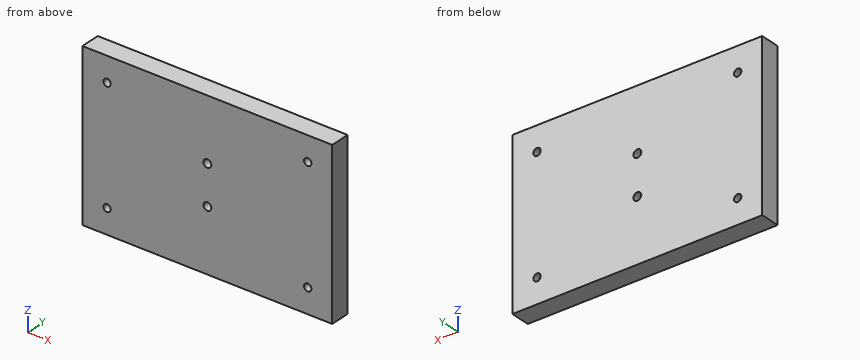
```python
from build123d import *

# Parameters (mm, degrees)
F0_W     = 101.69682
F0_H     = 66.800862
F1_DEPTH = 4
F3_D     = 3
F4_D     = 3.2


with BuildPart() as f1:
    # F0 (on Front) → F1 (new body, symmetric)
    with BuildSketch(Plane.XZ):
        Rectangle(F0_W, F0_H)
    extrude(amount=F1_DEPTH, both=True)

    # F3 (through all)
    with Locations(Plane.XZ.offset(4)):
        with Locations((-40.84841, 23.400431), (40.84841, 23.400431), (40.84841, -23.400431), (-40.84841, -23.400431)):
            Hole(F3_D / 2)

    # F4 (through all)
    with Locations(Plane.XZ.offset(4)):
        with Locations((0, 8), (0, -8)):
            Hole(F4_D / 2)


solid = f1.part
```
Input: part model. Units: mm. Frame: model coordinates. Coordinates: 2 decimals unless noted, no trailing zeros. Loops run counter-clockwise (first coordinate to the right, second up) from the corner with the lowest first, then second, coordinate; pieces in that order, holes last. Notation, with made-up numbers: M -37.75,27 L 14.25,27 A23 ccw 14.25,46 Z; hole C 73,-34 d5. An arc over 180 degrees is marked long. Use a Markdown table: item, result. Add a question column.
1) Section B-B, the plane x = 0. Return the cut outline in (y, z).
2) Line query: L1, parallel to Z at x = 0, y = 2; L2, parallel to X at y = 2, z = 23; L3, parallel to X at y = 3.5, z = -7. Output: solid intervals per line, ascending. Write a range as from..to.
3) Section A-A, the plane z = 8. Return the cut outline in (x, y).
4) Pin query (flat end, axial travel): P1, Ø3.5, axis at x = 0, z = 8, coming from the +Y side. Return the tip coordinate at first contact, or that it passes through.
Answer below:
| question | item | result |
|---|---|---|
| 1 | outline | M -4,-33.4 L 4,-33.4 L 4,-9.6 L -4,-9.6 Z; M -4,-6.4 L 4,-6.4 L 4,6.4 L -4,6.4 Z; M -4,9.6 L 4,9.6 L 4,33.4 L -4,33.4 Z |
| 2 | L1 | -33.4..-9.6, -6.4..6.4, 9.6..33.4 |
| 2 | L2 | -50.85..-42.29, -39.4..39.4, 42.29..50.85 |
| 2 | L3 | -50.85..-1.25, 1.25..50.85 |
| 3 | outline | M -50.85,-4 L -1.6,-4 L -1.6,4 L -50.85,4 Z; M 1.6,-4 L 50.85,-4 L 50.85,4 L 1.6,4 Z |
| 4 | P1 | y = 4 |
